```python
from build123d import *

# Parameters (mm, degrees)
SKETCH1_W           = 40
SKETCH1_H           = 40
BOSS_EXTRUDE1_DEPTH = 5
SKETCH2_R           = 1.25
CUT_EXTRUDE1_DEPTH  = 5
CIRPATTERN1_COUNT   = 4
SKETCH3_R           = 1.5
CUT_EXTRUDE3_DEPTH  = 10


with BuildPart() as part:
    # Sketch1 → Boss-Extrude1 (new body)
    with BuildSketch(Plane(origin=(0, 0, 0), x_dir=(1, 0, 0), z_dir=(0, 1, 0))):
        Rectangle(SKETCH1_W, SKETCH1_H)
    extrude(amount=BOSS_EXTRUDE1_DEPTH)

    # Sketch2 → Cut-Extrude1 (cut)
    with BuildSketch(Plane.XY.offset(20)):
        with Locations((-10, 2.5)):
            Circle(SKETCH2_R)
        with Locations(Location((10, 2.5, 0), (0, 0, 180))):
            Circle(SKETCH2_R)
    cut_extrude1 = extrude(amount=-CUT_EXTRUDE1_DEPTH, mode=Mode.SUBTRACT)

    # CirPattern1: Cut-Extrude1 ×4 about axis
    cirpattern1_axis = Axis((0, 0, 0), (0, 1, 0))
    for i in range(1, CIRPATTERN1_COUNT):
        add(cut_extrude1.rotate(cirpattern1_axis, i * 360 / CIRPATTERN1_COUNT), mode=Mode.SUBTRACT)

    # Sketch3 → Cut-Extrude3 (cut)
    with BuildSketch(Plane(origin=(0, 5, 0), x_dir=(1, 0, 0), z_dir=(0, 1, 0))):
        with Locations(Location((-15, 15, 0), (0, 0, 270))):
            Circle(SKETCH3_R)
        with Locations(Location((15, 15, 0), (0, 0, 270))):
            Circle(SKETCH3_R)
        with Locations(Location((15, -15, 0), (0, 0, 270))):
            Circle(SKETCH3_R)
        with Locations(Location((-15, -15, 0), (0, 0, 270))):
            Circle(SKETCH3_R)
    extrude(amount=-CUT_EXTRUDE3_DEPTH, mode=Mode.SUBTRACT)


solid = part.part
```
The listing builds one solid part. Answer for the finished solid, in the listing's coordinates (mm). A direction names the side the tool comes from. Coordinates: 2 decimals unless noted, no trailing zeros. Order: outer loops, then holes, each group sorted by start corner. A loop starts at its lowest first (then second) coordinate and runs counter-clockwise, first axis right, second up. Notation, with made-up numbers: M -13.5,-11 L 43.5,-11 A30 cw 43.5,23 Z; hole C -3,15.5 d9. An arc over 180 degrees is marked long. Answer as a JSON object with one key per item and string values. Group by question number.
1. Section A-A on z = 10.5 is taken. Write down the section's boundary in (x, y), then the cut area to 3 significant figures.
2. Determine the mould class of faces 1 (the flat face through (0, 5, 0)), 2 (the flat face through (-20, 2, 0)), 3 (the cylindrical face through (11.25, 2.55, -17.54)) for opening direction X: released by +X, released by -X, zero draft, split by the parting line, or undercut.
3. A tool of negligible diameter and unlimited length cuts with its end or side. For faces 4 (the flat face through (-10, 3, 15)), 5 (the flat face through (-15, 2, 10)), 6 (the cylindrical face through (17.54, 2.55, 11.25)), 7 (the flat face through (-10, 2, -15)), from which of +Z, -Z, +X, -X, +Y, -Y can it reach the whole face along a straight path? Write none if from no direction.
4. Flat-ended cylindrical pins translate along their axes: P1, Ø1.5, axis at x = 10, y = 2.5, coming from the -Z side; P2, Ø2, axis at y = 2.5, z = 10, coming from the +X side; P3, Ø2, axis at x = -10, y = 2.5, coming from the +Z side. Find the tip coordinate at first contact, or state that the pin passes through.
5. Straight lines are drawn through the part: line 1 (X direction, y = 1.4, z = -18); line 2 (Y direction, x = 10, z = -16); line 3 (X direction, y = 3.85, z = 14). For each, find the intervals that lie inside material, in ascending order.
6. Section B-B on y = 2.5 is taken. State how many separate pieces and enclosed holes the cut face has, then the cut area to 3 significant figures.
Values follow:
{
 "1": {"outline": "M -20,0 L 20,0 L 20,1.35 L 15,1.35 L 15,3.65 L 20,3.65 L 20,5 L -20,5 L -20,3.65 L -15,3.65 L -15,1.35 L -20,1.35 Z", "area": "177 mm2"},
 "2": {"face 1": "zero draft", "face 2": "released by -X", "face 3": "undercut"},
 "3": {"face 4": "+Z", "face 5": "-X", "face 6": "+X", "face 7": "-Z"},
 "4": {"P1": "z = -15", "P2": "x = 15", "P3": "z = 15"},
 "5": {"line 1": "-20 to -10.59, -9.41 to 9.41, 10.59 to 20", "line 2": "0 to 1.25, 3.75 to 5", "line 3": "-20 to -16.12, -13.88 to 13.88, 16.12 to 20"},
 "6": {"separate pieces": "1", "enclosed holes": "4", "area": "1,470 mm2"}
}
